Input: part model. Units: mm. Frame: model coordinates. A direction names the side the tool comes from. Coordinates: 2 decimals unless noted, no trailing zeros. Write each loop counter-clockwise with the first axis right and the second up, starting at its lowest first coordinate (ties: lowest second). Pieces come first, ordered by that corner, then holes. Notation, with made-up numbers: M 28,35.25 L 58,35.25 A20 ccw 58,72.25 Z; hole C 62.25,1 d5. An arc over 180 degrees is marked long. Write each question's results on one line, items separated by ' | '. Start each with the question number.
1. Section query A-A, the plane x = -15. Output: boundary loops of the cut face in (y, z) (3 decimals), and give its area (3 significant figures).
2. Section query C-C, the plane x = -9.5. Output: boundary loops of the cut face in (y, z).
3. Set-up query: faces 1 (the flat face through (-0.35, 102.233, 7.605)), 2 (the flat face through (0, 111, 0)). Return all of +Z, -Z, +X, -X, +Y, -Y with unobstructed straight access to the full face (end or side cutting, diameter ignored); none if empty.
4. Section query D-D, the plane z = 10.75. Output: boundary loops of the cut face in (x, y), and give its area (3 significant figures).
5. Ray query, probe 1 along X at (y, z) = (104.25, -0.25); probe 2 along Z at (x, y) = (15, 106); probe 3 along X at (y, z) = (108, 2.25). Return the intervals inside material, ascending.
6. Section query B-B, the plane y = 107.75. Output: boundary loops of the cut face in (x, z).
7. Pull-direction query (Z, two-part tool) for faces 3 (the flat face through (0, 106, 15)), 4 (the flat face through (-25, 107, 0)), 5 (the flat face through (-0.35, 102.27, -7.4)); classes: +Z half, -Z half, draft (parallel to the pull), parting line (faces both ways), or undercut.
8. First-contact query: pin 1 (4 mm diameter, centred on x = 15, z = 0, fed in from +Y); pin 2 (6 mm diameter, centred on x = -6.5, z = 8.5, fed in from -Y); pin 3 (8 mm diameter, centred on x = 2, z = 5.5, fed in from -Y); pin 4 (2 mm diameter, centred on x = -9, z = 0, fed in from -Y). Flat tips, straight axial feed; report the tip coordinate or a pass-through.
```python
from build123d import *

# Parameters (mm, degrees)
SKETCH_2_W                  = 50
SKETCH_2_H                  = 30
EXTRUDE_1_DEPTH             = 6
HOLE_WIZARD_M81_D           = 6.8
HOLE_WIZARD_M81_CSINK_D     = 8.05
HOLE_WIZARD_M81_CSINK_ANGLE = 90
CUT_EXTRUDE_1_DEPTH         = 115.764977236
CUT_EXTRUDE_1_DEPTH_BACK    = 115.764977236


with BuildPart() as part:
    # Эскиз2 → Бобышка-Вытянуть1 (new, symmetric)
    with BuildSketch(Plane(origin=(0, 105, 0), x_dir=(1, 0, 0), z_dir=(0, 1, 0))):
        Rectangle(SKETCH_2_W, SKETCH_2_H)
    extrude(amount=EXTRUDE_1_DEPTH, both=True)

    # Отверстие обработанное метчиком M81 (through all)
    with Locations(Plane(origin=(0, 111, 0), x_dir=(1, 0, 0), z_dir=(0, 1, 0))):
        with Locations((15, 0), (-15, 0)):
            CounterSinkHole(HOLE_WIZARD_M81_D / 2, HOLE_WIZARD_M81_CSINK_D / 2, counter_sink_angle=HOLE_WIZARD_M81_CSINK_ANGLE)

    # Эскиз5 → Вырез-Вытянуть1 (cut, two sides: drawn at the far end of the back side and taken through both)
    with BuildSketch(Plane(origin=(0, 0, 0), x_dir=(0, 0, -1), z_dir=(1, 0, 0)).offset(-CUT_EXTRUDE_1_DEPTH_BACK)):
        Polygon((-34.027690918, 97.573514412), (0, 103.573514412), (34.027690918, 97.573514412), align=None)
    extrude(amount=CUT_EXTRUDE_1_DEPTH + CUT_EXTRUDE_1_DEPTH_BACK, mode=Mode.SUBTRACT)


solid = part.part
```
Answer:
1) outline: M 100.929,-15 L 111,-15 L 111,-4.025 L 110.375,-3.4 L 102.974,-3.4 Z; M 100.929,15 L 102.974,3.4 L 110.375,3.4 L 111,4.025 L 111,15 Z | area: 210 mm^2
2) outline: M 100.93,-15 L 111,-15 L 111,15 L 100.93,15 L 103.57,0 Z
3) face 1: +X, -X, -Y | face 2: +Z, -Z, +X, -X, +Y
4) outline: M -25,101.68 L 25,101.68 L 25,111 L -25,111 Z | area: 466 mm^2
5) probe 1: -25 to -18.39, -11.61 to 11.61, 18.39 to 25 | probe 2: -15 to -3.4, 3.4 to 15 | probe 3: -25 to -17.55, -12.45 to 12.45, 17.55 to 25
6) outline: M -25,-15 L 25,-15 L 25,15 L -25,15 Z; hole C -15,0 d6.8; hole C 15,0 d6.8
7) face 3: +Z half | face 4: draft | face 5: undercut
8) pin 1: through | pin 2: y = 101.55 | pin 3: y = 101.9 | pin 4: y = 103.4
